Source: three-view drawing plus pictorial views. Frame: mm from the lowest corner of the part. A direction names the side the tool comes from. Give positions to 0.01 mm unless a question says otherwise; leave off trailing zeros. Write each loop counter-clockwise with the first axis right and the second up, starting at its lowest first coordinate (ties: lowest second). Pieces come first, ordered by that corner, then holes.
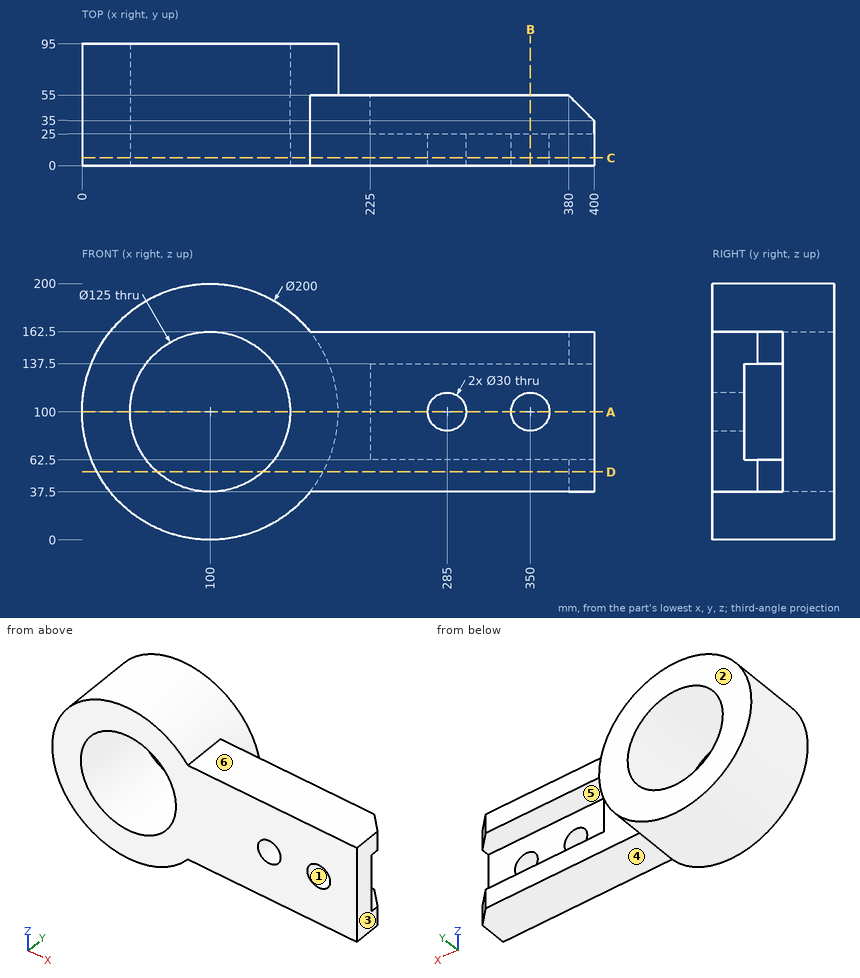
Q1. Pull-direction query (X, two-part tool) for the marked faces 1, 2 and 3; classes: released by +X, released by -X, zero draft, split by the parting line, or undercut.
Filled sheet:
face 1: undercut
face 2: zero draft
face 3: released by +X
Q2. Ray query, line 1 along X through (y, z) = (12.75, 100); line 2 along Z through (x, y) = (323.5, 26); line 3 along Z through (x, y) = (282.5, 16). Return the intervals inside material, ascending.
Filled sheet:
line 1: x = 0 to 37.5, 162.5 to 270, 300 to 335, 365 to 400
line 2: z = 37.5 to 62.5, 137.5 to 162.5
line 3: z = 37.5 to 85.21, 114.79 to 162.5
Q3. Pin query (flat end, axial travel): P1, Ø24, axis at y = 42, z = 113.5, coming from the +X side; P2, Ø1.5, axis at y = 22.5, z = 113, coming from the -X side; P3, Ø10, axis at x = 81, y = 55.5, coming from the -Z side. Return the tip coordinate at first contact, or that it passes through.
Filled sheet:
P1: stops at x = 225
P2: stops at x = 0.75
P3: stops at z = 0.98
Q4. Section A-A on z = 100. Output: boundary loops of the cut face in (x, y).
Filled sheet:
outline: (0, 0) - (37.5, 0) - (37.5, 95) - (0, 95) - close; (162.5, 0) - (270, 0) - (270, 25) - (225, 25) - (225, 55) - (200, 55) - (200, 95) - (162.5, 95) - close; (300, 0) - (335, 0) - (335, 25) - (300, 25) - close; (365, 0) - (400, 0) - (400, 25) - (365, 25) - close
Q5. Section B-B on x = 350. Output: boundary loops of the cut face in (y, z).
Filled sheet:
outline: (0, 37.5) - (55, 37.5) - (55, 62.5) - (25, 62.5) - (25, 85) - (0, 85) - close; (0, 115) - (25, 115) - (25, 137.5) - (55, 137.5) - (55, 162.5) - (0, 162.5) - close
Q6. Access query for the marked faces 4, 5 and 6. Directions: +Z, -Z, +X, -X, +Y, -Y. A direction counts if a zero-diameter tool reaches every point of the face in a straight line with its end or side. Return the directions, or none.
Filled sheet:
face 4: -Z, +X, +Y, -Y
face 5: +X, +Y
face 6: +Z, +X, +Y, -Y
Q7. Section D-D on z = 53. Output: boundary loops of the cut face in (x, y), plus the area to 3 significant figures.
Filled sheet:
outline: (11.73, 0) - (58.8, 0) - (58.8, 95) - (11.73, 95) - close; (141.2, 0) - (400, 0) - (400, 35) - (380, 55) - (188.27, 55) - (188.27, 95) - (141.2, 95) - close
area: 20,400 mm2
Q8. Section C-C on y = 6. Output: boundary loops of the cut face in (x, z), plus the area to 3 significant figures.
Filled sheet:
outline: (178.06, 37.5) - (400, 37.5) - (400, 162.5) - (178.06, 162.5) arc R100 ccw (long way) to start; hole circle Ø125 at (100, 100); hole circle Ø30 at (285, 100); hole circle Ø30 at (350, 100)
area: 43,600 mm2
